Autodesk Inventor part; units mm, degrees
ref_plane "YZ Plane" through (0, 0, 0) normal (1, 0, 0) x (0, 1, 0)
ref_plane "XZ Plane" through (0, 0, 0) normal (0, 1, 0) x (-1, 0, 0)
ref_plane "XY Plane" through (0, 0, 0) normal (0, 0, 1) x (1, 0, 0)
sketch "Sketch1" plane through (0, 0, 0) normal (0, 1, 0) x (-1, 0, 0)
  line L0 (-37.465, -32.512) -> (37.465, -32.512)
  line L1 (37.465, -32.512) -> (37.465, 32.512)
  line L2 (37.465, 32.512) -> (-37.465, 32.512)
  line L3 (-37.465, 32.512) -> (-37.465, -32.512)
  line L4 (-37.465, -32.512) -> (37.465, 32.512) construction
  line L5 (37.465, -32.512) -> (-37.465, 32.512) construction
  point P0 (0, 0)
  point P1 (0, 0)
  dimension "d0" = 74.93
  dimension "d1" = 65.024
extrude "Extrusion1" add sketch "Sketch1" along normal blind 25.654
sketch "Sketch2" plane through (-37.465, 0, 32.512) normal (0, 0, 1) x (1, 0, 0)
  line L0 (74.93, 0) -> (74.93, 25.654)
  line L1 (0, 25.654) -> (74.93, 25.654)
  line L2 (0, 0) -> (0, 25.654)
  circle A0 centre (37.465, 16.764) radius 3.175
  point P0 (37.465, 0)
  dimension "d4" = 6.35
  dimension "d5" = 37.465
  dimension "d6" = 37.465
  dimension "d7" = 8.89
extrude "Extrusion2" cut sketch "Sketch2" against normal blind 5.588
sketch "Sketch3" plane through (-37.465, 0, 32.512) normal (0, 0, 1) x (1, 0, 0)
  circle A0 centre (37.465, 16.764) radius 3.175
  line L0 (74.93, 0) -> (74.93, 25.654)
  line L1 (0, 0) -> (0, 25.654)
  circle A1 centre (57.531, 16.764) radius 1.143
  line L2 (37.465, 25.654) -> (37.465, 0) construction
  circle A2 centre (17.399, 16.764) radius 1.143
  dimension "d10" = 2.286
  dimension "d11" = 20.066
  dimension "d12" = 20.066
  dimension "d13" = 37.465
  dimension "d14" = 37.465
extrude "Extrusion3" cut sketch "Sketch3" against normal blind 4.318 contours A1 | A2
ref_plane "Work Plane1" through (-37.465, 0, 0) normal (0, 0, 1) x (1, 0, 0)
mirror "Mirror1" about plane through (-37.465, 0, 0) normal (0, 0, 1) of "Extrusion2", "Extrusion3"
ref_plane "Work Plane2" through (0, 0, 32.512) normal (1, 0, 0) x (0, 0, -1)
sketch "Sketch4" plane through (37.465, 0, 32.512) normal (1, 0, 0) x (0, 0, -1)
  line L0 (0, 25.654) -> (65.024, 25.654)
  circle A0 centre (32.512, 16.6624) radius 3.175
  circle A1 centre (47.6004, 16.6624) radius 1.016
  line L1 (32.512, 25.654) -> (32.512, 0) construction
  circle A2 centre (17.4236, 16.6624) radius 1.016
  dimension "d19" = 6.35
  dimension "d20" = 8.9916
  dimension "d21" = 2.032
extrude "Extrusion4" cut sketch "Sketch4" against normal blind 4.318
mirror "Mirror2" about plane through (0, 0, 32.512) normal (1, 0, 0) of "Extrusion4"
sketch "Sketch5" plane through (0, 25.654, 0) normal (0, 1, 0) x (1, 0, 0)
  circle A0 centre (0, 0) radius 12.319
  dimension "d24" = 24.638
extrude "Extrusion5" cut sketch "Sketch5" against normal blind 8.636
sketch "Sketch6" plane through (37.465, 0, 32.512) normal (1, 0, 0) x (0, 0, -1)
  line L0 (0, 25.654) -> (65.024, 25.654)
  line L1 (25.2146, 11.43) -> (39.4386, 11.43)
  line L2 (39.4386, 11.43) -> (39.4386, 1.27)
  line L3 (39.4386, 1.27) -> (25.2146, 1.27)
  line L4 (25.2146, 1.27) -> (25.2146, 11.43)
  point P0 (32.512, 0)
  dimension "d27" = 14.224
  dimension "d28" = 10.16
  dimension "d29" = 14.224
extrude "Extrusion6" add sketch "Sketch6" along normal blind 1.016
sketch "Sketch7" plane through (38.481, 0, 32.512) normal (1, 0, 0) x (0, 0, -1)
  line L0 (25.2146, 11.43) -> (25.2146, 1.27)
  line L1 (39.4386, 1.27) -> (39.4386, 11.43)
  line L2 (26.8656, 8.4177) -> (37.7876, 8.4177)
  line L3 (37.7876, 8.4177) -> (37.7876, 2.5757)
  line L4 (37.7876, 2.5757) -> (26.8656, 2.5757)
  line L5 (26.8656, 4.6339) -> (26.8656, 6.3596)
  line L6 (26.8656, 4.6339) -> (29.2737, 2.5757)
  line L7 (26.8656, 5.4967) -> (37.7876, 5.4967) construction
  line L8 (26.8656, 6.3596) -> (29.2737, 8.4177)
  point P0 (32.512, 0)
  dimension "d32" = 5.842
  dimension "d34" = 10.922
  dimension "d35" = 1.651
  dimension "d36" = 1.651
extrude "Extrusion7" cut sketch "Sketch7" against normal blind 7.62
fillet "Fillet1" radius 3.175 12 edges at (0, 25.654, -32.512) (37.465, 12.827, -32.512) (37.465, 25.654, 0) (-37.465, 25.654, 0) (-37.465, 12.827, -32.512) (0, 0, -32.512) (37.465, 0, 0) (-37.465, 0, 0) (0, 0, 32.512) (37.465, 12.827, 32.512) (0, 25.654, 32.512) (-37.465, 12.827, 32.512)
equation "\"d5\" = d6"
equation "\"d12\" = d11"
equation "\"d13\" = d14"
equation "\"d35\" = d36"
properties part number "dragonfly2Camera" material "Aluminum 6061"
Geometry: final body of the model. Coordinates: model frame, mm. A direction names the side the tool comes from. Round coordinates to 2 decimals unless told otherwise and drop trailing zeros. Loops run counter-clockwise (first coordinate to the right, second up) from the corner with the lowest first, then second, coordinate; pieces in that order, holes last. Notation, with made-up numbers: (7, 26) -> (58, 26) arc R29 cw to (58, 58) -> close; hole circle Ø5 at (65.25, 46.5). An arc over 180 degrees is marked (long way). Write each question's results on one line, items separated by ' | '.
Item 1: Set-up query: faces 1 (the face through (34.72, 3.62, 4.46)), 2 (the face through (38, 1.27, 0)), 3 (the face through (21.156, 17.107, 30.383)). Return all of +Z, -Z, +X, -X, +Y, -Y with unobstructed straight access to the full face (end or side cutting, diameter ignored); none if empty.
Answers below:
face 1: +X | face 2: +Z, -Z, +X, -Y | face 3: +Z
Item 2: Cut plane C-C on y = 14.5. Return the cut outline in (x, z) (3 decimals).
Answers below:
outline: (-37.465, -29.337) arc R3.175 ccw to (-34.29, -32.512) -> (-2.226, -32.512) -> (-2.226, -26.924) -> (2.226, -26.924) -> (2.226, -32.512) -> (34.29, -32.512) arc R3.175 ccw to (37.465, -29.337) -> (37.465, -2.325) -> (33.147, -2.325) -> (33.147, 2.325) -> (37.465, 2.325) -> (37.465, 29.337) arc R3.175 ccw to (34.29, 32.512) -> (2.226, 32.512) -> (2.226, 26.924) -> (-2.226, 26.924) -> (-2.226, 32.512) -> (-34.29, 32.512) arc R3.175 ccw to (-37.465, 29.337) -> (-37.465, 2.325) -> (-33.147, 2.325) -> (-33.147, -2.325) -> (-37.465, -2.325) -> close
Item 3: Cut plane A-A on z = 19. Return the cut outline in (x, y) (3 decimals).
Answers below:
outline: (-37.465, 3.175) arc R3.175 ccw to (-34.29, 0) -> (34.29, 0) arc R3.175 ccw to (37.465, 3.175) -> (37.465, 22.479) arc R3.175 ccw to (34.29, 25.654) -> (-34.29, 25.654) arc R3.175 ccw to (-37.465, 22.479) -> close
Item 4: Cut plane B-B on x = 0. Return the cut outline in (y, z) (3 decimals), and give its area (3 significant figures).
Answers below:
outline: (0, -29.337) arc R3.175 ccw to (3.175, -32.512) -> (13.589, -32.512) -> (13.589, -26.924) -> (19.939, -26.924) -> (19.939, -32.512) -> (22.479, -32.512) arc R3.175 ccw to (25.654, -29.337) -> (25.654, -12.319) -> (17.018, -12.319) -> (17.018, 12.319) -> (25.654, 12.319) -> (25.654, 29.337) arc R3.175 ccw to (22.479, 32.512) -> (19.939, 32.512) -> (19.939, 26.924) -> (13.589, 26.924) -> (13.589, 32.512) -> (3.175, 32.512) arc R3.175 ccw to (0, 29.337) -> close | area: 1,380 mm²
Item 5: Pin query (flat end, axial travel): pin 1 Ø1.3 at (x, y) = (37.5, 6) entering from -Z; pin 2 Ø1.5 at (y, z) = (5, -25.5) entering from +X (3 decimals); pin 3 Ø0.5 at (x, z) = (37.5, 1) entering from -Y. Return the tip coordinate at first contact, or that it passes through.
Answers below:
pin 1: stops at z = -31.22 | pin 2: stops at x = 37.465 | pin 3: stops at y = 1.27
Item 6: Line query: probe 1 along Y at (x, z) = (0, -29.35); probe 2 along Z at (x, y) = (0, 22.25); probe 3 along Y at (x, z) = (-4.5, 5). Output: solid intervals per line, ascending. Write a range as [from, to].
Answers below:
probe 1: y = [0, 13.59], [19.94, 25.65] | probe 2: z = [-32.51, -12.32], [12.32, 32.51] | probe 3: y = [0, 17.02]
Item 7: Pull-direction query (Z, two-part tool) for faces 4 (the face through (-2.671, 21.396, 12.026)), 5 (the face through (36.56, 12.692, 31.557)), 6 (the face through (-36.56, 24.7, -0.41)); classes: pulls with the +Z half, pulls with the -Z half, needs draft (parallel to the pull), parting line crosses it, or undercut.
Answers below:
face 4: undercut | face 5: pulls with the +Z half | face 6: needs draft
Item 8: Cut plane D-D on z = 0. Return the cut outline in (x, y) (3 decimals), and give its area (3 significant figures).
Answers below:
outline: (-37.465, 3.175) arc R3.175 ccw to (-34.29, 0) -> (34.29, 0) arc R3.175 ccw to (36.83, 1.27) -> (38.481, 1.27) -> (38.481, 2.576) -> (30.861, 2.576) -> (30.861, 8.418) -> (38.481, 8.418) -> (38.481, 11.43) -> (37.465, 11.43) -> (37.465, 13.487) -> (33.147, 13.487) -> (33.147, 19.837) -> (37.465, 19.837) -> (37.465, 22.479) arc R3.175 ccw to (34.29, 25.654) -> (12.319, 25.654) -> (12.319, 17.018) -> (-12.319, 17.018) -> (-12.319, 25.654) -> (-34.29, 25.654) arc R3.175 ccw to (-37.465, 22.479) -> (-37.465, 19.837) -> (-33.147, 19.837) -> (-33.147, 13.487) -> (-37.465, 13.487) -> close | area: 1,610 mm²
